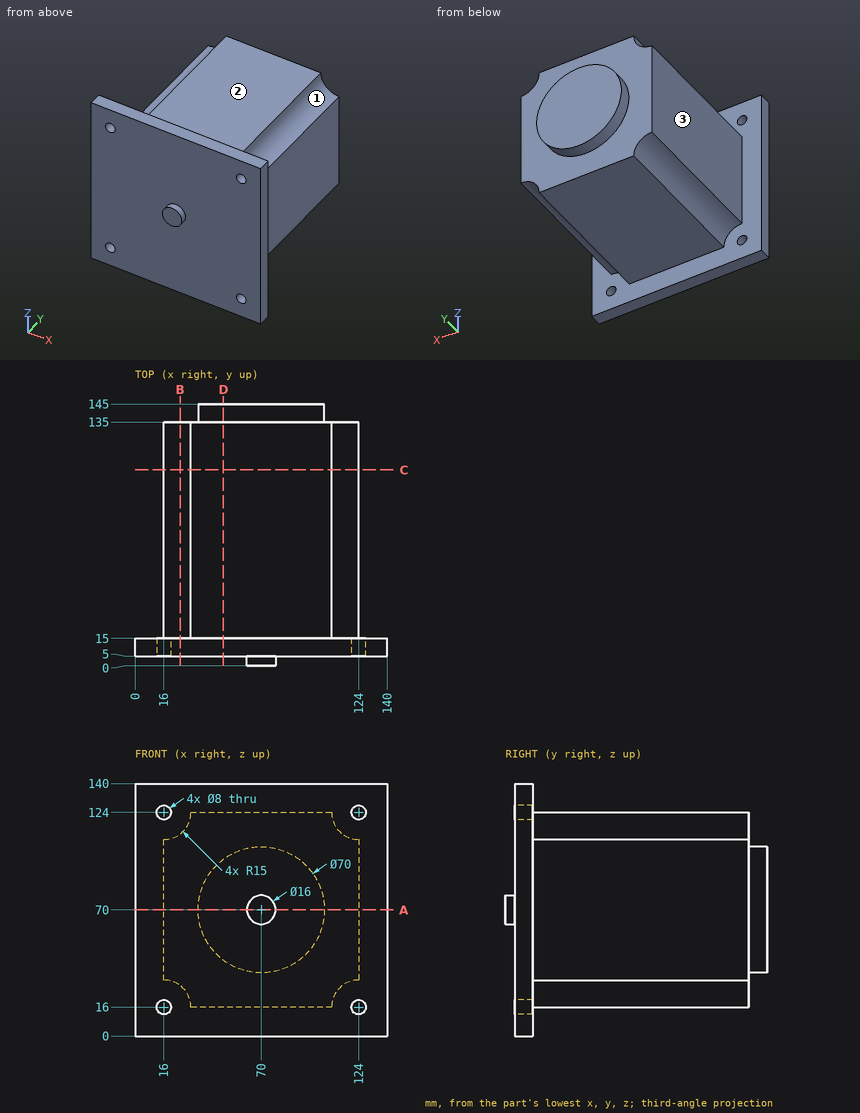
Part print with two shaded views. Sizes in mm from the minimum x, y, z corner. A direction names the side the tool comes from. Round coordinates to 2 decimals unless told otherwise and drop trailing zeros. Write each loop counter-clockwise with the first axis right and the second up, starting at its lowest first coordinate (ties: lowest second). Pieces come first, ordered by that corner, then holes. Notation, with made-up numbers: (37, 23.5) -> (79, 23.5) arc R18 ccw to (79, 47.5) -> close; hole circle Ø8 at (8, -2.75). An arc over 180 degrees is marked (long way). Use one line per item in the form item = value.
Q1. Tool access for the marked faces 1, 2 and 3: list every direction of +Z, -Z, +X, -X, +Y, -Y with a clear straight run to the whole face (end or side of a thin tool).
Conclusion:
face_1 = +Z, +X, +Y
face_2 = +Z, +X, -X, +Y
face_3 = +Z, -Z, -X, +Y
Q2. Band-saw the part on B-B, the plane x = 25. Write the cut outline in (y, z).
Conclusion:
outline = (5, 0) -> (15, 0) -> (15, 28) -> (135, 28) -> (135, 112) -> (15, 112) -> (15, 140) -> (5, 140) -> close
Q3. Band-saw the part on A-A, the plane z = 70. Write the cut outline in (x, y).
Conclusion:
outline = (0, 5) -> (62, 5) -> (62, 0) -> (78, 0) -> (78, 5) -> (140, 5) -> (140, 15) -> (124, 15) -> (124, 135) -> (105, 135) -> (105, 145) -> (35, 145) -> (35, 135) -> (16, 135) -> (16, 15) -> (0, 15) -> close
Q4. Band-saw the part on C-C, the plane y = 108.5. Write the cut outline in (x, z).
Conclusion:
outline = (16, 31) arc R15 cw to (31, 16) -> (109, 16) arc R15 cw to (124, 31) -> (124, 109) arc R15 cw to (109, 124) -> (31, 124) arc R15 cw to (16, 109) -> close
Q5. Drop flat-ended pins along their axis: P1, Ø12, axis at y = 130, z = 45, coming from the +X side; P2, Ø1, axis at x = 106.5, z = 66.5, coming from the +Y side; P3, Ø9, axis at x = 16, z = 16, coming from the +Y side; P4, Ø7, axis at x = 124, z = 124, coming from the -Y side. Give the stop position or say it passes through.
Conclusion:
P1 = 124
P2 = 135
P3 = 15
P4 = through
Q6. Drill centre lines: L1, parallel to Z at x = 124, y = 13.25; L2, parallel to Y at x = 113, z = 100. Where is each one in solid material? Low to high.
Conclusion:
L1 = 0 to 12, 20 to 120, 128 to 140
L2 = 5 to 135
Q7. Band-saw the part on D-D, the plane x = 49. Write the cut outline in (y, z).
Conclusion:
outline = (5, 0) -> (15, 0) -> (15, 16) -> (135, 16) -> (135, 42) -> (145, 42) -> (145, 98) -> (135, 98) -> (135, 124) -> (15, 124) -> (15, 140) -> (5, 140) -> close
